Can you work these out from the model? Positions are in its coordinate system, mm. A direction names the side the tool comes from. Coordinates: 2 decimals unless noted, no trailing zeros. Loops run counter-clockwise (first coordinate to the right, second up) from the corner with the lowest first, then second, coordinate; pieces in that order, holes last. Notation, with made-up numbers: (71.25, -29.5) - (112.25, -29.5) arc R17 cw to (112.25, -13.5) - close; hole circle Ø9 at (49, 17.5). An arc over 180 degrees is marked (long way). Put each result on its own line as item: value. Start each with the question number.
from build123d import *

# Parameters (mm, degrees)
F0_R         = 12.7
F1_DEPTH     = 1.5875
F2_R         = 11.1125
F3_DEPTH     = 8
F4_W         = 25.4
F4_H         = 25.4
F5_DEPTH     = 6.35
F6_R         = 2.5
F7_DEPTH     = 15.9375
F8_R         = 1.5875
F9_REACH     = 29.8911280605
F10_T1_DEPTH = 69.85


# Not quite as in the source:
# - a fillet or chamfer that OpenCascade refuses, or shapes differently, is made with other operations: its cross-section is extruded or revolved along the edge and cut away or added


with BuildPart() as f1:
    # F0 (on Top) → F1 (new body)
    with BuildSketch(Plane.XY):
        Circle(F0_R)
    extrude(amount=F1_DEPTH)

    # F2 (on face) → F3 (join)
    with BuildSketch(Plane.XY.offset(1.5875)):
        Circle(F2_R)
    extrude(amount=F3_DEPTH)

    # F4 (on face) → F5 (join)
    with BuildSketch(Plane.XY.offset(9.5875)):
        Rectangle(F4_W, F4_H)
    extrude(amount=F5_DEPTH)

    # F6 (on face) → F7 (cut, through all)
    with BuildSketch(Plane.XY.offset(15.9375)):
        Circle(F6_R)
    extrude(amount=-F7_DEPTH, mode=Mode.SUBTRACT)

    f9_end = f1.faces().sort_by_distance((-2.5, 0, 7.96875))[0]
    # F8 (on face) → F9 (cut, up to a face of the model that its end follows)
    with BuildSketch(Plane(origin=(0, 12.7, 0), x_dir=(-1, 0, 0), z_dir=(0, 1, 0))):
        with Locations((0, 12.7625)):
            Circle(F8_R)
    f9_long = extrude(amount=-F9_REACH, mode=Mode.PRIVATE)
    add(split(f9_long, bisect_by=f9_end, keep=Keep.ALL, mode=Mode.PRIVATE).solids().sort_by_distance((0, 12.7, 12.7625))[0], mode=Mode.SUBTRACT)

    # F10: fillet of radius 12.7 on 4 edges, made by hand

    # F10_s2 → F10_t1 (cut)
    with BuildSketch(Plane.XY.offset(-22.1625)):
        with BuildLine():
            ThreePointArc((-12.7, 0), (-8.9802561211, 8.9802561211), (0, 12.7))
            Line((0, 12.7), (-12.7, 12.7))
            Line((-12.7, 12.7), (-12.7, 0))
        make_face()
        with BuildLine():
            ThreePointArc((0, -12.7), (-8.9802561211, -8.9802561211), (-12.7, 0))
            Line((-12.7, 0), (-12.7, -12.7))
            Line((-12.7, -12.7), (0, -12.7))
        make_face()
        with BuildLine():
            ThreePointArc((12.7, 0), (8.9802561211, 8.9802561211), (0, 12.7))
            Line((0, 12.7), (12.7, 12.7))
            Line((12.7, 12.7), (12.7, 0))
        make_face()
        with BuildLine():
            ThreePointArc((0, -12.7), (8.9802561211, -8.9802561211), (12.7, 0))
            Line((12.7, 0), (12.7, -12.7))
            Line((12.7, -12.7), (0, -12.7))
        make_face()
    extrude(amount=F10_T1_DEPTH, mode=Mode.SUBTRACT)


solid = f1.part
Q1. I want a section at A-A on y = 3.75. List the corners of the cut face in (x, z) for me (1 decimal).
Q2. Will these pins go through, and if not, where does the flat tip stop? pin 1 (4 mm diameter, centred on y = -1.5, z = 2.5, fed in from +X); pin 2 (8 mm diameter, centred on x = 3.5, z = 6.5, fed in from -Y); pin 3 (2 mm diameter, centred on x = -6.5, z = 7.5, fed in from +Y); pin 4 (1.5 mm diameter, centred on x = -1.5, z = 9, fed in from +Y).
Q3. On a 3-axis mill with a long thin cutter (end or side, diameter ignored), from which of +Z, -Z, +X, -X, +Y, -Y can I reach the whole of each face in a straight line? I mean faces 5 (the cylindrical face through (-0.54, -2.44, 8.08)), 6 (the flat face through (0.88, -11.23, 9.588)). Say none if no direction works.
Q4. Please list where these lines run through material, in increasing order: line 1 along Y through (x, z) = (0, 4.25); line 2 along Z through (x, y) = (-7.25, 9.25); line 3 along Y through (x, z) = (0, 9.75). Write a range as [from, to].
Q5. I want a section at D-D on y = -9.25. List the corners of the cut face in (x, z) for me, and give its area (3 significant figures).
Q6. I want a section at C-C on x = -7.25. List the corners of the cut face in (y, z) for me.
Q7. I want a section at B-B on z = 10.75. List the corners of the cut face in (x, y) for me, and give its area (3 significant figures).
Q8. We'd pull the mould along Z, two halves only. Please class faces 1 (the cylindrical face through (0.207, 7.391, 14.336)), 2 (the cylindrical face through (-2.75, -12.4, 0.78)), 3 (the flat face through (0.88, -11.23, 1.588)), 4 (the flat face through (3, 0, 15.938)): released by +Z, released by -Z, zero draft, split by the parting line, or undercut.
Calculated:
1. outline: (-12.1, 0) - (12.1, 0) - (12.1, 1.6) - (10.5, 1.6) - (10.5, 9.6) - (12.1, 9.6) - (12.1, 15.9) - (-12.1, 15.9) - (-12.1, 9.6) - (-10.5, 9.6) - (-10.5, 1.6) - (-12.1, 1.6) - close; hole circle Ø3.2 at (0, 12.8)
2. pin 1: x = 12.7
2. pin 2: y = -12.66
2. pin 3: y = 9.66
2. pin 4: y = 12.66
3. face 5: +Z, -Z
3. face 6: none
4. line 1: [-11.11, -2.5], [2.5, 11.11]
4. line 2: [0, 1.59], [9.59, 15.94]
4. line 3: [-12.7, -2.5], [2.5, 12.7]
5. outline: (-8.7, 0) - (8.7, 0) - (8.7, 1.59) - (6.16, 1.59) - (6.16, 9.59) - (8.7, 9.59) - (8.7, 15.94) - (-8.7, 15.94) - (-8.7, 9.59) - (-6.16, 9.59) - (-6.16, 1.59) - (-8.7, 1.59) - close
5. area: 237 mm2
6. outline: (-10.43, 0) - (10.43, 0) - (10.43, 1.59) - (8.42, 1.59) - (8.42, 9.59) - (10.43, 9.59) - (10.43, 15.94) - (-10.43, 15.94) - (-10.43, 9.59) - (-8.42, 9.59) - (-8.42, 1.59) - (-10.43, 1.59) - close
7. outline: circle Ø25.4 at (0, 0); hole circle Ø5 at (0, 0)
7. area: 487 mm2
8. face 1: undercut
8. face 2: zero draft
8. face 3: undercut
8. face 4: released by +Z
